from build123d import *

# Parameters (mm, degrees)
SKETCH1_W            = 16.6
SKETCH1_H            = 20
BOSS_EXTRUDE1_DEPTH  = 2
EXTRUDE_THIN1_DEPTH  = 0.5
SKETCH3_R            = 2.875
BOSS_EXTRUDE2_DEPTH  = 0.5
M4_CLEARANCE_HOLE1_D = 4.5
DEBURS_SIZE          = 0.2


with BuildPart() as part:
    # Sketch1 → Boss-Extrude1 (new body)
    with BuildSketch(Plane.XY):
        Rectangle(SKETCH1_W, SKETCH1_H)
    extrude(amount=-BOSS_EXTRUDE1_DEPTH)

    # Sketch2 → Extrude-Thin1 (add)
    with BuildSketch(Plane.XY):
        Polygon((8.3, 10), (-8.3, 10), (-8.3, -10), (8.3, -10), (8.3, -7.6), (-5.9, -7.6), (-5.9, 7.6), (8.3, 7.6), align=None)
    extrude(amount=EXTRUDE_THIN1_DEPTH)

    # Sketch3 → Boss-Extrude2 (add)
    with BuildSketch(Plane.XY):
        with Locations(Location((0, 0, 0), (0, 0, 180))):
            Circle(SKETCH3_R)
    extrude(amount=BOSS_EXTRUDE2_DEPTH)

    # M4 Clearance Hole1 (through all)
    with Locations(Plane(origin=(0, 0, -2), x_dir=(-1, 0, 0), z_dir=(0, 0, -1))):
        with Locations((0, 0)):
            Hole(M4_CLEARANCE_HOLE1_D / 2)

    # Deburs
    deburs_edges = [part.edges().sort_by_distance(p)[0] for p in [
        (-8.3, 0, -2),
        (8.3, 0, 0),
        (8.3, -8.8, 0.5),
        (1.2, -7.6, 0.5),
        (0, -10, -2),
        (8.3, -7.6, 0.25),
        (-5.9, 0, 0.5),
        (1.2, 7.6, 0.5),
        (8.3, 8.8, 0.5),
        (8.3, 7.6, 0.25),
        (0, -10, 0.5),
        (0, 10, 0.5),
        (-8.3, 0, 0.5),
        (2.875, 0, 0.5),
        (-2.25, 0, -2),
        (-2.25, 0, 0.5),
        (8.3, 0, -2),
        (8.3, -10, -0.75),
        (-8.3, -10, -0.75),
        (-8.3, 10, -0.75),
        (8.3, 10, -0.75),
        (0, 10, -2),
    ]]
    chamfer(deburs_edges, length=DEBURS_SIZE)


solid = part.part
The listing builds one solid part. Answer for the finished solid, in the listing's coordinates (mm). A direction names the side the tool comes from. Give positions to 0.01 mm unless a question says otherwise; leave off trailing zeros. Order: outer loops, then holes, each group sorted by start corner. A loop starts at its lowest first (then second) coordinate and runs counter-clockwise, first axis right, second up. Notation, with made-up numbers: (-33.75, -29) - (-3.75, -29) arc R9 ccw to (-3.75, -17) - close; hole circle Ø7 at (4, -34). An arc over 180 degrees is marked (long way). One line per item, written item: value. Start each with the question number.
1) A cutting plane is placed at A-A on y = 0. Give the vertices of the cut face in (x, z) (3 decimals).
2) A cutting plane is placed at C-C on z = -0.55. Give the vertices of the cut face in (x, y), then the cut area to 3 significant figures.
3) A tool of negligible diameter and unlimited length cuts with its end or side. For faces 4 (the face through (0.37, -2.85, 0.15)), 5 (the face through (-8.3, 0, -1)), from which of +Z, -Z, +X, -X, +Y, -Y can it reach the whole face along a straight path? Write none if from no direction.
4) The mould has two halves that part along Y. Classify faces 1 (the face through (-0.29, 2.23, -0.74)), 2 (the face through (-2, 2, -2)), 3 (the face through (0, 10, -1)): released by +Y, released by -Y, zero draft, split by the parting line, or undercut.
5) A cutting plane is placed at D-D on y = -7. Give the vertices of the cut face in (x, z).
6) Given pin 1 Ø1.5 at (x, y) = (3.5, -4) entering from +Z; pin 2 Ø7 at (x, y) = (0, 0) entering from +Z, each flat-ended and moving along its own axis, determine where each tip first touches the part or whether it passes through.
7) Find the intervals of material crossed by L1, parallel to Y at x = 6, z = 0.1; L2, parallel to Y at x = 0, z = -0.6; L3, parallel to X at y = -1, z = 0.2, in increasing order.
8) A cutting plane is placed at B-B on x = 0. Give the vertices of the cut face in (y, z) (3 decimals), then the cut area to 3 significant figures.
Answer sheet:
1. outline: (-8.3, -1.8) - (-8.1, -2) - (-2.45, -2) - (-2.25, -1.8) - (-2.25, 0.3) - (-2.45, 0.5) - (-2.675, 0.5) - (-2.875, 0.3) - (-2.875, 0) - (-5.9, 0) - (-5.9, 0.3) - (-6.1, 0.5) - (-8.1, 0.5) - (-8.3, 0.3) - close; (2.25, -1.8) - (2.45, -2) - (8.1, -2) - (8.3, -1.8) - (8.3, -0.2) - (8.1, 0) - (2.875, 0) - (2.875, 0.3) - (2.675, 0.5) - (2.45, 0.5) - (2.25, 0.3) - close
2. outline: (-8.3, -9.8) - (-8.1, -10) - (8.1, -10) - (8.3, -9.8) - (8.3, 9.8) - (8.1, 10) - (-8.1, 10) - (-8.3, 9.8) - close; hole circle Ø4.5 at (0, 0)
2. area: 316 mm2
3. face 4: +Z
3. face 5: +Z, -Z, -X, +Y, -Y
4. face 1: undercut
4. face 2: zero draft
4. face 3: released by +Y
5. outline: (-8.3, -1.8) - (-8.1, -2) - (8.1, -2) - (8.3, -1.8) - (8.3, -0.2) - (8.1, 0) - (-5.9, 0) - (-5.9, 0.3) - (-6.1, 0.5) - (-8.1, 0.5) - (-8.3, 0.3) - close
6. pin 1: stops at z = 0
6. pin 2: stops at z = 0.5
7. L1: y = -10 to -7.6, 7.6 to 10
7. L2: y = -10 to -2.25, 2.25 to 10
7. L3: x = -8.3 to -5.9, -2.7 to -2.02, 2.02 to 2.7
8. outline: (-10, -1.8) - (-9.8, -2) - (-2.45, -2) - (-2.25, -1.8) - (-2.25, 0.3) - (-2.45, 0.5) - (-2.675, 0.5) - (-2.875, 0.3) - (-2.875, 0) - (-7.6, 0) - (-7.6, 0.3) - (-7.8, 0.5) - (-9.8, 0.5) - (-10, 0.3) - close; (2.25, -1.8) - (2.45, -2) - (9.8, -2) - (10, -1.8) - (10, 0.3) - (9.8, 0.5) - (7.8, 0.5) - (7.6, 0.3) - (7.6, 0) - (2.875, 0) - (2.875, 0.3) - (2.675, 0.5) - (2.45, 0.5) - (2.25, 0.3) - close
8. area: 33.8 mm2
